Build history of the part. All positions in model axes, mm. Face numbers are marked on the shaded views. A direction names the side the tool comes from. Round coordinates to 2 decimals unless told otherwise and drop trailing zeros. Loops run counter-clockwise (first coordinate to the right, second up) from the corner with the lowest first, then second, coordinate; pieces in that order, holes last. Notation, with made-up numbers: M 12,58.25 L 47,58.25 A35 cw 47,95.25 Z; hole C 80,67 d7. An arc over 180 degrees is marked long. One line per item, written item: value.
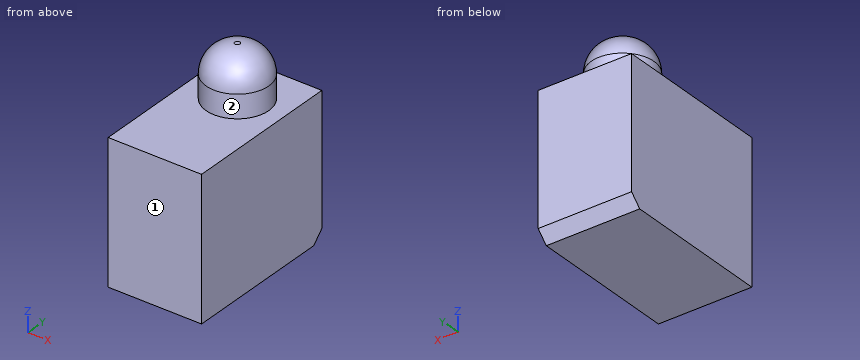
```python
from build123d import *

# Parameters (mm, degrees)
BOSS_EXTRUDE1_DEPTH      = 2.16
BOSS_EXTRUDE1_DEPTH_BACK = 2.16
SKETCH1_W                = 6.5
SKETCH1_H                = 7.4
SKETCH2_R                = 1.45
BOSS_EXTRUDE2_DEPTH      = 2.4
FILLET1_R                = 1.33
CHAMFER1_SIZE            = 0.5


with BuildPart() as part:
    # Sketch1 → Boss-Extrude1 (new, two sides: drawn at the far end of the back side and taken through both)
    with BuildSketch(Plane(origin=(0, 0, 0), x_dir=(0, 0, -1), z_dir=(1, 0, 0)).offset(-BOSS_EXTRUDE1_DEPTH_BACK)):
        Rectangle(SKETCH1_W, SKETCH1_H)
    extrude(amount=BOSS_EXTRUDE1_DEPTH + BOSS_EXTRUDE1_DEPTH_BACK)

    # Sketch2 → Boss-Extrude2 (add)
    with BuildSketch(Plane.XY.offset(3.25)):
        with Locations((0, 1.38)):
            Circle(SKETCH2_R)
    extrude(amount=BOSS_EXTRUDE2_DEPTH)

    # Fillet1
    fillet1_edges = [part.edges().sort_by_distance(p)[0] for p in [
        (-1.45, 1.38, 5.65),
    ]]
    fillet(fillet1_edges, radius=FILLET1_R)

    # Chamfer1
    chamfer1_edges = [part.edges().sort_by_distance(p)[0] for p in [
        (0, 3.7, -3.25),
    ]]
    chamfer(chamfer1_edges, length=CHAMFER1_SIZE)


solid = part.part
```
Item 1: Slice it at A-A, the plane z = 4. Give the cut face in (x, y), and give its area (3 significant figures).
Check values:
outline: C 0,1.38 d2.9
area: 6.61 mm2
Item 2: Drop a flat-ended pin along its axis: P1, Ø1.5, axis at x = -1, y = 0.5, coming from the +Z side. Give the stop position or say it passes through.
Check values:
P1: stops at z = 5.57
Item 3: Slice it at B-B, the plane y = -2. Give the cut face in (x, z), and give its area (3 significant figures).
Check values:
outline: M -2.16,-3.25 L 2.16,-3.25 L 2.16,3.25 L -2.16,3.25 Z
area: 28.1 mm2
Item 4: Which spindle directions (+Z, -Z, +X, -X, +Y, -Y) get a long thin tool onto all of the face, cutting with end or side? Do the marked faces 1 and 2. Say none if no direction does.
Check values:
face 1: +Z, -Z, +X, -X, -Y
face 2: +Z
Item 5: Wall check: line 1 along Z through (x, y) = (1.5, -0.75); line 2 along Y through (x, z) = (-0.6, 5.25); line 3 along Z through (x, y) = (-0.95, 0.5). Give the ranges that are in metal, low to high.
Check values:
line 1: z = -3.25 to 3.25
line 2: y = 0.49 to 2.27
line 3: z = -3.25 to 4.94
